Could you check a few things on this model? Use its own coordinates, in mm. Give positions to 0.01 mm unless a question says otherwise; leave off trailing zeros. Write each loop counter-clockwise with the first axis right and the second up, starting at its lowest first coordinate (ties: lowest second). Pieces come first, ordered by that corner, then holes. Notation, with made-up numbers: (20, 21) - (27, 21) arc R22 ccw to (27, 54) - close; hole circle Ø2 at (-22, -15). An arc over 180 degrees is marked (long way). Write item = value, one per line.
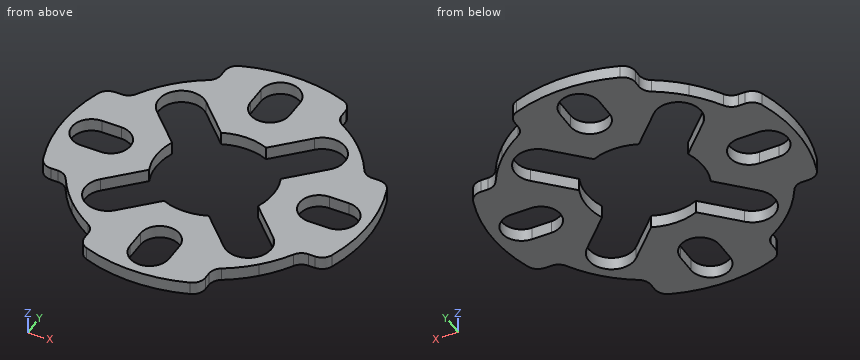
from build123d import *

# Parameters (mm, degrees)
F1_DEPTH = 1


with BuildPart() as f1:
    # F0 (on Top) → F1 (new body)
    with BuildSketch(Plane.XY):
        with BuildLine():
            ThreePointArc((4.64256, 10.16719), (4.460262, 10.742831), (3.979834, 11.108597))
            ThreePointArc((3.979834, 11.108597), (0, 11.8), (-3.979834, 11.108597))
            ThreePointArc((-3.979834, 11.108597), (-4.460262, 10.742831), (-4.64256, 10.16719))
            Line((-4.64256, 10.16719), (-4.64256, 9.633))
            ThreePointArc((-4.64256, 9.633), (-4.774969, 9.135722), (-5.137132, 8.770131))
            ThreePointArc((-5.137132, 8.770131), (-6.21269, 8.044117), (-7.186979, 7.186979))
            ThreePointArc((-7.186979, 7.186979), (-8.044117, 6.21269), (-8.770131, 5.137132))
            ThreePointArc((-8.770131, 5.137132), (-9.135722, 4.774969), (-9.633, 4.64256))
            Line((-9.633, 4.64256), (-10.16719, 4.64256))
            ThreePointArc((-10.16719, 4.64256), (-10.742831, 4.460262), (-11.108597, 3.979834))
            ThreePointArc((-11.108597, 3.979834), (-11.8, 0), (-11.108597, -3.979834))
            ThreePointArc((-11.108597, -3.979834), (-10.742831, -4.460262), (-10.16719, -4.64256))
            Line((-10.16719, -4.64256), (-9.633, -4.64256))
            ThreePointArc((-9.633, -4.64256), (-9.135722, -4.774969), (-8.770131, -5.137132))
            ThreePointArc((-8.770131, -5.137132), (-8.044117, -6.21269), (-7.186979, -7.186979))
            ThreePointArc((-7.186979, -7.186979), (-6.21269, -8.044117), (-5.137132, -8.770131))
            ThreePointArc((-5.137132, -8.770131), (-4.774969, -9.135722), (-4.64256, -9.633))
            Line((-4.64256, -9.633), (-4.64256, -10.16719))
            ThreePointArc((-4.64256, -10.16719), (-4.460262, -10.742831), (-3.979834, -11.108597))
            ThreePointArc((-3.979834, -11.108597), (0, -11.8), (3.979834, -11.108597))
            ThreePointArc((3.979834, -11.108597), (4.460262, -10.742831), (4.64256, -10.16719))
            Line((4.64256, -10.16719), (4.64256, -9.633))
            ThreePointArc((4.64256, -9.633), (4.774969, -9.135722), (5.137132, -8.770131))
            ThreePointArc((5.137132, -8.770131), (6.21269, -8.044117), (7.186979, -7.186979))
            ThreePointArc((7.186979, -7.186979), (8.044117, -6.21269), (8.770131, -5.137132))
            ThreePointArc((8.770131, -5.137132), (9.135722, -4.774969), (9.633, -4.64256))
            Line((9.633, -4.64256), (10.16719, -4.64256))
            ThreePointArc((10.16719, -4.64256), (10.742831, -4.460262), (11.108597, -3.979834))
            ThreePointArc((11.108597, -3.979834), (11.8, 0), (11.108597, 3.979834))
            ThreePointArc((11.108597, 3.979834), (10.742831, 4.460262), (10.16719, 4.64256))
            Line((10.16719, 4.64256), (9.633, 4.64256))
            ThreePointArc((9.633, 4.64256), (9.135722, 4.774969), (8.770131, 5.137132))
            ThreePointArc((8.770131, 5.137132), (8.044117, 6.21269), (7.186979, 7.186979))
            ThreePointArc((7.186979, 7.186979), (6.21269, 8.044117), (5.137132, 8.770131))
            ThreePointArc((5.137132, 8.770131), (4.774969, 9.135722), (4.64256, 9.633))
            Line((4.64256, 9.633), (4.64256, 10.16719))
        make_face()
        with BuildLine():
            ThreePointArc((-9.5, -1.5), (-11, 0), (-9.5, 1.5))
            Line((-9.5, 1.5), (-8, 1.5))
            ThreePointArc((-8, 1.5), (-6.5, 0), (-8, -1.5))
            Line((-8, -1.5), (-9.5, -1.5))
        make_face(mode=Mode.SUBTRACT)
        with BuildLine():
            Line((1.5, -8), (1.5, -9.5))
            ThreePointArc((1.5, -9.5), (0, -11), (-1.5, -9.5))
            Line((-1.5, -9.5), (-1.5, -8))
            ThreePointArc((-1.5, -8), (0, -6.5), (1.5, -8))
        make_face(mode=Mode.SUBTRACT)
        with BuildLine():
            Line((-4.17097, 6.596394), (-1.729112, 4.154536))
            ThreePointArc((-1.729112, 4.154536), (0, 4.5), (1.729112, 4.154536))
            Line((1.729112, 4.154536), (4.17097, 6.596394))
            ThreePointArc((4.17097, 6.596394), (6.65805, 6.584305), (6.621784, 4.097461))
            Line((6.621784, 4.097461), (4.183111, 1.658788))
            ThreePointArc((4.183111, 1.658788), (4.5, 0), (4.183111, -1.658788))
            Line((4.183111, -1.658788), (6.621784, -4.097461))
            ThreePointArc((6.621784, -4.097461), (6.65805, -6.584305), (4.17097, -6.596394))
            Line((4.17097, -6.596394), (1.729112, -4.154536))
            ThreePointArc((1.729112, -4.154536), (0, -4.5), (-1.729112, -4.154536))
            Line((-1.729112, -4.154536), (-4.17097, -6.596394))
            ThreePointArc((-4.17097, -6.596394), (-6.65805, -6.584305), (-6.621784, -4.097461))
            Line((-6.621784, -4.097461), (-4.183111, -1.658788))
            ThreePointArc((-4.183111, -1.658788), (-4.5, 0), (-4.183111, 1.658788))
            Line((-4.183111, 1.658788), (-6.621784, 4.097461))
            ThreePointArc((-6.621784, 4.097461), (-6.65805, 6.584305), (-4.17097, 6.596394))
        make_face(mode=Mode.SUBTRACT)
        with BuildLine():
            Line((8, 1.5), (9.5, 1.5))
            ThreePointArc((9.5, 1.5), (11, 0), (9.5, -1.5))
            Line((9.5, -1.5), (8, -1.5))
            ThreePointArc((8, -1.5), (6.5, 0), (8, 1.5))
        make_face(mode=Mode.SUBTRACT)
        with BuildLine():
            ThreePointArc((-1.5, 9.5), (0, 11), (1.5, 9.5))
            Line((1.5, 9.5), (1.5, 8))
            ThreePointArc((1.5, 8), (0, 6.5), (-1.5, 8))
            Line((-1.5, 8), (-1.5, 9.5))
        make_face(mode=Mode.SUBTRACT)
    extrude(amount=F1_DEPTH)


solid = f1.part
1. For pin 1 (0.5 mm diameter, centred on y = 9, z = 0.5, fed in from +X), with a flat end and sliding along its axis, tell me the tip position at first contact or that it passes through.
Filled sheet:
pin_1 = 5.17
2. If we section it at C-C, the plane y = -6: Please give me the cut outline in (x, z), and give its area (3 significant figures).
Filled sheet:
outline = (-8.2, 0) - (-7.04, 0) - (-7.04, 1) - (-8.2, 1) - close; (-3.57, 0) - (3.57, 0) - (3.57, 1) - (-3.57, 1) - close; (7.04, 0) - (8.2, 0) - (8.2, 1) - (7.04, 1) - close
area = 9.48 mm2
3. If we section it at A-A, the plane x = 0: Please give me the cut outline in (y, z), and give its area (3 significant figures).
Filled sheet:
outline = (-11.8, 0) - (-11, 0) - (-11, 1) - (-11.8, 1) - close; (-6.5, 0) - (-4.5, 0) - (-4.5, 1) - (-6.5, 1) - close; (4.5, 0) - (6.5, 0) - (6.5, 1) - (4.5, 1) - close; (11, 0) - (11.8, 0) - (11.8, 1) - (11, 1) - close
area = 5.60 mm2
4. I need wall thicknesses on line 1 (X direction, y = 6.75, z = 0.2); line 2 (Y direction, x = -5.5, z = 0.4); line 3 (X direction, y = -6, z = 0.3). Which ranges of each line are inside material? Lowest first, please.
Filled sheet:
line_1 = -7.6 to -6.47, -4.35 to -0.83, 0.83 to 4.35, 6.47 to 7.6
line_2 = -8.55 to -7.11, -2.98 to 2.98, 7.11 to 8.55
line_3 = -8.2 to -7.04, -3.57 to 3.57, 7.04 to 8.2
5. If we section it at D-D, the plane y = 7.5: Please give me the cut outline in (x, z).
Filled sheet:
outline = (-6.86, 0) - (-1.41, 0) - (-1.41, 1) - (-6.86, 1) - close; (1.41, 0) - (6.86, 0) - (6.86, 1) - (1.41, 1) - close
